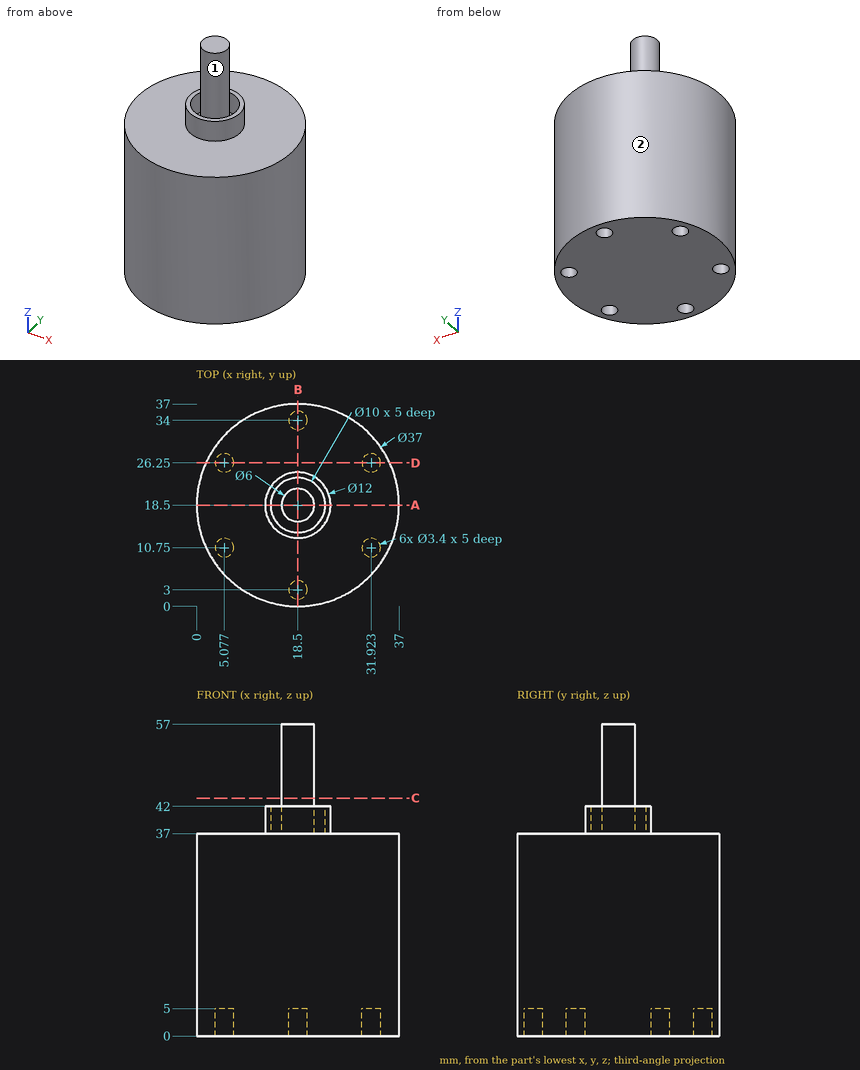
Drawing for the job (mm, zero at the part's lowest x, y, z). A direction names the side the tool comes from. Give positions to 0.01 mm unless a question says otherwise; leave off trailing zeros. Order: outer loops, then holes, each group sorted by start corner. A loop starts at its lowest first (then second) coordinate and runs counter-clockwise, first axis right, second up. Notation, with made-up numbers: M 17,81.5 L 65,81.5 A20 cw 65,118.5 Z; hole C -3.5,45 d7. An arc over 180 degrees is marked long. Put each result on its own line as item: value. Start each with the question number.
(1) Saw through at B-B, the plane x = 18.5. Write the cut outline in (y, z), then the cut area to 4 significant figures.
(2) Saw through at D-D, the plane y = 26.25. Write the cut outline in (x, z), then the cut area to 3 significant figures.
(3) Saw through at C-C, the plane z = 43.5. Write the cut outline in (x, y).
(4) Which spindle directions (+Z, -Z, +X, -X, +Y, -Y) get a long thin tool onto all of the face, cutting with end or side? Do the marked faces 1 and 2. Say none if no direction does.
(5) Drill centre lines: line 1 along Y through (x, z) = (18.5, 1.2); line 2 along Y through (x, z) = (18.5, 38.05); line 3 along X through (y, z) = (26, 2) (1 decimal). Where is each one in solid material? Low to high.
(6) Flat gauge pins, fed straight in: pin 1 Ø4 at (x, y) = (18.5, 34) entering from -Z; pin 2 Ø2.5 at (x, y) = (5.08, 26.25) entering from +Z; pin 3 Ø1 at (x, y) = (19.5, 2.5) entering from -Z; pin 4 Ø1 at (y, z) = (11.5, 6.5) entering from +X. Where does each tip first touch, or does it go through?
(7) Saw through at A-A, the plane y = 18.5. Write the cut outline in (x, z).
Check result:
1. outline: M 0,0 L 1.3,0 L 1.3,5 L 4.7,5 L 4.7,0 L 32.3,0 L 32.3,5 L 35.7,5 L 35.7,0 L 37,0 L 37,37 L 24.5,37 L 24.5,42 L 23.5,42 L 23.5,37 L 21.5,37 L 21.5,57 L 15.5,57 L 15.5,37 L 13.5,37 L 13.5,42 L 12.5,42 L 12.5,37 L 0,37 Z
1. area: 1,465 mm2
2. outline: M 1.7,0 L 3.38,0 L 3.38,5 L 6.78,5 L 6.78,0 L 30.22,0 L 30.22,5 L 33.62,5 L 33.62,0 L 35.3,0 L 35.3,37 L 1.7,37 Z
2. area: 1,210 mm2
3. outline: C 18.5,18.5 d6
4. face 1: +Z
4. face 2: +Z, -Z
5. line 1: y = 0 to 1.3, 4.7 to 32.3, 35.7 to 37
5. line 2: y = 12.5 to 13.5, 15.5 to 21.5, 23.5 to 24.5
5. line 3: x = 1.6 to 3.4, 6.8 to 30.2, 33.6 to 35.4
6. pin 1: stops at z = 0
6. pin 2: stops at z = 37
6. pin 3: stops at z = 5
6. pin 4: stops at x = 35.82
7. outline: M 0,0 L 37,0 L 37,37 L 24.5,37 L 24.5,42 L 23.5,42 L 23.5,37 L 21.5,37 L 21.5,57 L 15.5,57 L 15.5,37 L 13.5,37 L 13.5,42 L 12.5,42 L 12.5,37 L 0,37 Z
